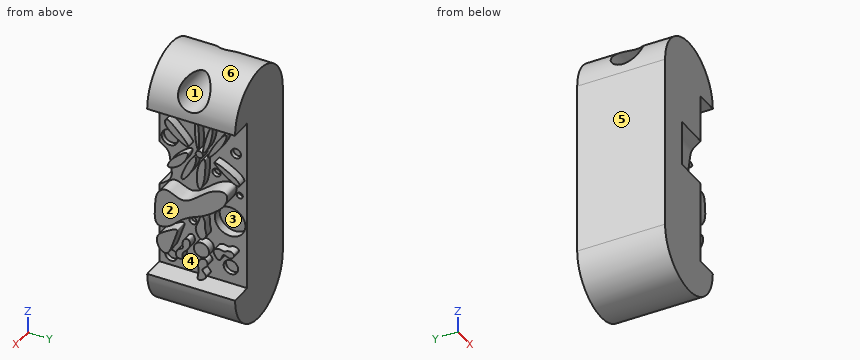
from build123d import *

# Parameters (mm, degrees)
F0_W      = 18.9466625452
F0_H      = 50.8
F1_DEPTH  = 25.4
F3_DEPTH  = 2.54
F5_DEPTH  = 2.54
F7_DEPTH  = 2.54
F9_DEPTH  = 2.54
F10_R     = 2.2037661108
F11_DEPTH = 2.54
F13_DEPTH = 2.54
F14_R     = 1.0473543245
F15_DEPTH = 2.54
F16_R     = 4.4029393082
F17_DEPTH = 2.54
F19_DEPTH = 5.08
F21_DEPTH = 3.81
F22_R     = 1.460983402
F22_R_2   = 0.8761261726
F22_R_3   = 1.1998887947
F22_R_4   = 2.3822273237
F22_R_5   = 0.7813065252
F22_R_6   = 1.0693889774
F22_R_7   = 2.0974618181
F22_R_8   = 1.7434208878
F23_DEPTH = 1.27
F25_DEPTH = 10
F26_R     = 4.1855782258
F27_DEPTH = 30
F28_R     = 4.3688404115
F29_DEPTH = 30


with BuildPart() as f1:
    # F0 (on Front) → F1 (new body)
    with BuildSketch(Plane.XZ):
        with Locations((9.4733312726, 25.4)):
            Rectangle(F0_W, F0_H)
        with BuildLine():
            ThreePointArc((25.4, 50.8), (12.7, 63.5), (0, 50.8))
            Line((0, 50.8), (18.9466625452, 50.8))
            Line((18.9466625452, 50.8), (25.4, 50.8))
        make_face()
        with BuildLine():
            Line((18.9466625452, 0), (0, 0))
            ThreePointArc((0, 0), (12.7, -12.7), (25.4, 0))
            Line((25.4, 0), (18.9466625452, 0))
        make_face()
    extrude(amount=F1_DEPTH)

    # F2 (on face) → F3 (join)
    with BuildSketch(Plane.YZ.offset(18.9466625452)):
        with BuildLine():
            add(Edge.make_bspline(
                [(-12.7, 0), (-12.1587068574, -0.186421223), (-9.1969725356, 1.6701898847), (-12.7819987666, 3.3689946826), (-9.2587764915, 5.0029186659), (-10.9635852494, 7.6674219674), (-13.3264466897, 5.3689109873), (-12.2777824387, 2.859032607), (-13.2255103376, 0.1809856289), (-12.7, 0)],
                knots=[0, 0, 0, 0, 0.1523574371, 0.2848373169, 0.4303792872, 0.5559419632, 0.6935722887, 0.852084939, 1, 1, 1, 1], degree=3))
        make_face()
    extrude(amount=F3_DEPTH)

    # F4 (on face) → F5 (join)
    with BuildSketch(Plane.YZ.offset(18.9466625452)):
        with BuildLine():
            add(Edge.make_bspline(
                [(-19.05, 5.1723495126), (-19.4676667532, 5.7480486345), (-18.8380971455, 7.7744991793), (-16.8329186801, 7.9006968747), (-17.7052345676, 10.2787269645), (-15.9676377207, 12.0297018569), (-14.713319284, 10.2458093106), (-15.8014853333, 7.9636604801), (-17.7105856123, 6.7550427596), (-16.9534289215, 4.4899133227), (-18.7043333124, 4.6958930865), (-19.05, 5.1723495126)],
                knots=[0, 0, 0, 0, 0.1239474728, 0.2239006727, 0.3401700303, 0.4492065796, 0.5476283947, 0.67433429, 0.7936623829, 0.8974193852, 1, 1, 1, 1], degree=3))
        make_face()
    extrude(amount=F5_DEPTH)

    # F6 (on face) → F7 (join)
    with BuildSketch(Plane.YZ.offset(18.9466625452)):
        with BuildLine():
            add(Edge.make_bspline(
                [(-12.0711624622, 12.7573236823), (-11.4367969336, 12.5809759526), (-9.930944509, 14.1377853484), (-11.0370818754, 16.2251107005), (-10.5445469328, 18.0899061765), (-11.9527375102, 21.2721387382), (-12.800618147, 16.9117405663), (-13.9329669541, 15.9171914125), (-12.8567334616, 12.9757051296), (-12.0711624622, 12.7573236823)],
                knots=[0, 0, 0, 0, 0.1357388721, 0.273513971, 0.4115631689, 0.5425887856, 0.7045688045, 0.8319068162, 1, 1, 1, 1], degree=3))
        make_face()
    extrude(amount=F7_DEPTH)

    # F8 (on face) → F9 (join)
    with BuildSketch(Plane.YZ.offset(18.9466625452)):
        with BuildLine():
            add(Edge.make_bspline(
                [(-8.3441883326, 10.1769361645), (-8.320056966, 10.9401703438), (-6.7873812738, 11.6821238495), (-5.342859624, 10.7781428021), (-4.1922333759, 11.9050739461), (-1.7399280852, 11.2243552708), (-3.4361736571, 8.6409088637), (-5.8925577474, 11.0342997762), (-6.2222248998, 6.4557549482), (-8.3734810962, 9.2504557541), (-8.3441883326, 10.1769361645)],
                knots=[0, 0, 0, 0, 0.1246108644, 0.2350107813, 0.3427220566, 0.461856938, 0.5834474213, 0.7127028173, 0.8487364325, 1, 1, 1, 1], degree=3))
        make_face()
    extrude(amount=F9_DEPTH)

    # F10 (on face) → F11 (join)
    with BuildSketch(Plane.YZ.offset(18.9466625452)):
        with Locations((-11.8481758982, 9.3916803598)):
            Circle(F10_R)
    extrude(amount=F11_DEPTH)

    # F12 (on face) → F13 (join)
    with BuildSketch(Plane.YZ.offset(18.9466625452)):
        with BuildLine():
            add(Edge.make_bspline(
                [(-15.9412715584, 37.8425680101), (-16.4599835343, 38.1529996788), (-19.891275436, 35.3347747815), (-20.9513538421, 33.8732644194), (-22.298560563, 31.2201488002), (-17.3643612808, 32.8414492587), (-15.3920591024, 37.51388283), (-15.9412715584, 37.8425680101)],
                knots=[0, 0, 0, 0, 0.2273545918, 0.403395234, 0.5422844026, 0.7592768635, 1, 1, 1, 1], degree=3))
        make_face()
        with BuildLine():
            add(Edge.make_bspline(
                [(-15.6496744603, 39.8572906852), (-15.1360683338, 40.208744889), (-19.7316768365, 45.124463423), (-22.2108583757, 47.079159636), (-23.0450446539, 43.6487662378), (-16.2102746602, 39.4736790287), (-15.6496744603, 39.8572906852)],
                knots=[0, 0, 0, 0, 0.3013413171, 0.4984679094, 0.6710864729, 1, 1, 1, 1], degree=3))
        make_face()
        with BuildLine():
            add(Edge.make_bspline(
                [(-13.093996793, 48.7732067704), (-13.3700980694, 49.3022797668), (-14.3216212376, 46.2645126057), (-12.1172625697, 34.2225792128), (-12.5600894495, 47.7501185698), (-13.093996793, 48.7732067704)],
                knots=[0, 0, 0, 0, 0.2168902151, 0.5805912956, 1, 1, 1, 1], degree=3))
        make_face()
        with BuildLine():
            add(Edge.make_bspline(
                [(-11.3084185869, 39.6522730589), (-11.6745395246, 40.0885909503), (-10.0499884165, 46.1826032552), (-8.3069572408, 50.0403093232), (-8.8120334679, 42.6215044235), (-11.0460895976, 39.3396473126), (-11.3084185869, 39.6522730589)],
                knots=[0, 0, 0, 0, 0.3096002981, 0.4918508665, 0.7781685643, 1, 1, 1, 1], degree=3))
        make_face()
        with BuildLine():
            add(Edge.make_bspline(
                [(-9.8847821355, 38.6147089303), (-10.2641676442, 38.8681195069), (-7.3475032709, 44.6080636696), (-4.0295370076, 48.3340183153), (-5.2681860616, 43.2176057853), (-9.5080921651, 38.3630988386), (-9.8847821355, 38.6147089303)],
                knots=[0, 0, 0, 0, 0.2865502063, 0.4982687259, 0.7154857362, 1, 1, 1, 1], degree=3))
        make_face()
        with BuildLine():
            add(Edge.make_bspline(
                [(-8.0946544185, 37.5679135323), (-7.5740868469, 37.8618887854), (-0.9790549856, 34.6530871044), (-0.5001687291, 31.7044634891), (-4.2698106136, 33.7033312857), (-8.5291807406, 37.3225275488), (-8.0946544185, 37.5679135323)],
                knots=[0, 0, 0, 0, 0.3310804974, 0.4899534876, 0.7236416582, 1, 1, 1, 1], degree=3))
        make_face()
        with BuildLine():
            add(Edge.make_bspline(
                [(-10.7293128967, 36.4189296961), (-10.6481049738, 34.8011686243), (-10.8525102266, 30.0190099959), (-12.9876015825, 26.5691960414), (-13.6573586062, 34.6039540936), (-10.9548430259, 38.2259802602), (-10.762670421, 37.0834523465), (-10.7293128967, 36.4189296961)],
                knots=[0, 0, 0, 0, 0.2744228725, 0.4222272432, 0.6882010074, 0.8872761759, 1, 1, 1, 1], degree=3))
        make_face()
        with BuildLine():
            add(Edge.make_bspline(
                [(-13.721363619, 37.5530123711), (-14.4497998914, 37.4682734483), (-17.5042396654, 32.1501550566), (-17.9086044815, 27.653236669), (-13.3059752224, 34.3446549325), (-13.2503910693, 37.6078005633), (-13.721363619, 37.5530123711)],
                knots=[0, 0, 0, 0, 0.3100138558, 0.4962902609, 0.7995596572, 1, 1, 1, 1], degree=3))
        make_face()
    extrude(amount=F13_DEPTH)

    # F14 (on face) → F15 (join)
    with BuildSketch(Plane.YZ.offset(18.9466625452)):
        with Locations((-12.4654732645, 38.6147387326)):
            Circle(F14_R)
    extrude(amount=F15_DEPTH)

    # F16 (on face) → F17 (cut)
    with BuildSketch(Plane.YZ.offset(18.9466625452)):
        with Locations((-4.9326894805, 18.8860446215)):
            Circle(F16_R)
    extrude(amount=-F17_DEPTH, mode=Mode.SUBTRACT)

    # F18 (on face) → F19 (join)
    with BuildSketch(Plane.YZ.offset(18.9466625452)):
        with BuildLine():
            add(Edge.make_bspline(
                [(-23.1685712934, 15.2417980134), (-22.3854114778, 14.6366031784), (-19.2684715864, 15.5490991832), (-16.9750424784, 18.5224602193), (-13.2351329617, 20.7209840815), (-9.9087599587, 21.6906775308), (-3.0723412858, 26.6384901245), (-2.6395408303, 31.9439683504), (-9.1287825512, 30.4097311386), (-15.3087659566, 22.8164756622), (-20.2874916771, 27.6106681471), (-23.6995879494, 25.0221215813), (-23.9248238363, 20.4016395773), (-24.1059658959, 15.9661793729), (-23.1685712934, 15.2417980134)],
                knots=[0, 0, 0, 0, 0.0711045703, 0.1476766262, 0.2244724336, 0.2979131955, 0.4080768304, 0.4786013556, 0.5641273371, 0.6777398914, 0.7629231677, 0.8300250604, 0.9148921598, 1, 1, 1, 1], degree=3))
        make_face()
    extrude(amount=F19_DEPTH)

    # F20 (on face) → F21 (join)
    with BuildSketch(Plane.YZ.offset(18.9466625452)):
        with BuildLine():
            add(Edge.make_bspline(
                [(-23.8294545561, 10.6006283313), (-23.4947747744, 11.4335393387), (-21.981735164, 12.4942936977), (-17.1763212025, 15.4872094726), (-19.2311995145, 10.912032711), (-20.621450181, 4.7573700994), (-24.0776370889, 7.4299235), (-24.1709015099, 9.7508759954), (-23.8294545561, 10.6006283313)],
                knots=[0, 0, 0, 0, 0.1532888673, 0.3271130329, 0.4885520691, 0.6973485205, 0.8436116561, 1, 1, 1, 1], degree=3))
        make_face()
    extrude(amount=F21_DEPTH)

    # F22 (on face) → F23 (cut)
    with BuildSketch(Plane.YZ.offset(18.9466625452)):
        with Locations((-3.2262913883, 40.4002405703)):
            Circle(F22_R)
        with Locations((-2.1561626345, 27.8180986643)):
            Circle(F22_R_2)
        with Locations((-8.8824778795, 32.6976887882)):
            Circle(F22_R_3)
        with Locations((-22.3465077579, 39.1590669751)):
            Circle(F22_R_4)
        with Locations((-18.1392524391, 49.5709590614)):
            Circle(F22_R_5)
        with Locations((-15.6395584345, 15.6808272004)):
            Circle(F22_R_6)
        with Locations((-4.7130216844, 4.9145147204)):
            Circle(F22_R_7)
        with Locations((-21.9584498554, 3.0254796147)):
            Circle(F22_R_8)
    extrude(amount=-F23_DEPTH, mode=Mode.SUBTRACT)

    # F24 (on face) → F25 (cut)
    with BuildSketch(Plane.YZ.offset(18.9466625452)):
        with BuildLine():
            add(Edge.make_bspline(
                [(-25.4, 36.9402728975), (-24.3854230216, 36.3314319699), (-22.2965318819, 35.0779026501), (-22.2658578991, 31.1301388709), (-21.1575912175, 26.5905444144), (-23.9638000112, 24.7904233309), (-25.4, 23.8691344857)],
                knots=[0, 0, 0, 0, 0.2297701488, 0.4730688801, 0.7303202362, 1, 1, 1, 1], degree=3))
            Line((-25.4, 36.9402728975), (-25.4, 23.8691344857))
        make_face()
    extrude(amount=-F25_DEPTH, mode=Mode.SUBTRACT)

    # F26 (on Right) → F27 (cut)
    with BuildSketch(Plane.YZ):
        with Locations((-12.6720517874, 58.0905079842)):
            Circle(F26_R)
    extrude(amount=-F27_DEPTH, mode=Mode.SUBTRACT)

    # F28 (on Right) → F29 (cut)
    with BuildSketch(Plane.YZ):
        with Locations((-13.0914794281, 57.9255223274)):
            Circle(F28_R)
    extrude(amount=F29_DEPTH, mode=Mode.SUBTRACT)


solid = f1.part
Part model, mm, in its own coordinate system. Face numbers are marked on the shaded views. A direction names the side the tool comes from. Give positions to 0.01 mm unless a question says otherwise; leave off trailing zeros. Loops run counter-clockwise (first coordinate to the right, second up) from the corner with the lowest first, then second, coordinate; pieces in that order, holes last. Notation, with made-up numbers: (21.25, 41.5) -> (29.25, 41.5) arc R21 cw to (29.25, 73.5) -> close; hole circle Ø1 at (23.5, 77.25). An arc over 180 degrees is marked (long way). Write each question's results on one line, items separated by ' | '. Start each with the question number.
Q1. Pin check, flat tips, straight feed: P1, Ø1.5, axis at x = 17, y = -7, coming from the -Z side; P2, Ø4.5, axis at y = -4.5, z = 5.5, coming from the +X side; P3, Ø6, axis at x = 19.5, y = -7.5, coming from the -Z side; P4, Ø4, axis at x = 12, y = -11, coming from the +Z side. Stop position of each tip, or through.
Q2. Which spindle directions (+Z, -Z, +X, -X, +Y, -Y) get a long thin tool onto all of the face, cutting with end or side? Do the marked faces 1, 2 and 3. Say none if no direction does.
Q3. Wall check: L1, parallel to Z at x = 19.5, y = -8.5; L2, parallel to X at y = -4.5, z = 38; L3, parallel to X at y = -1.5, z = 28. Give the ranges that are in metal, low to high.
Q4. Band-saw the part on A-A on z = 54.5. List the corners of the cut face in (x, y), plus the area to 3 significant figures.
Q5. Band-saw the part on C-C on z = -6.5. List the corners of the cut face in (x, y).
Q6. Band-saw the part on B-B on x = 4.5. List the corners of the cut face in (y, z), plus the area to 3 significant figures.
Q7. Pull direction Z, two halves, no side cores. Call the marked faces 4, 5 and 6: +Z half, -Z half, draft (parallel to the pull), parting line (faces both ways), or undercut.
Results are:
1) P1: stops at z = -12.19 | P2: stops at x = 18.95 | P3: stops at z = -12.12 | P4: stops at z = 63.5
2) face 1: +X, -X | face 2: +X, +Y, -Y | face 3: +X
3) L1: z = -10.73 to 0, 22.9 to 29.71, 39.71 to 42.1, 50.8 to 61.53 | L2: x = 0 to 18.95 | L3: x = 0 to 17.68
4) outline: (0.55, -25.4) -> (24.85, -25.4) -> (24.85, -15.8) -> (0.55, -15.8) -> close; (0.55, -10.38) -> (24.85, -10.38) -> (24.85, 0) -> (0.55, 0) -> close | area: 485 mm²
5) outline: (1.79, -25.4) -> (23.61, -25.4) -> (23.61, 0) -> (1.79, 0) -> close
6) outline: (-25.4, -9.7) -> (0, -9.7) -> (0, 60.5) -> (-9.56, 60.5) arc R4.37 cw (long way) to (-16.62, 60.5) -> (-25.4, 60.5) -> close | area: 1,730 mm²
7) face 4: undercut | face 5: draft | face 6: +Z half
